```python
from build123d import *

# Parameters (mm, degrees)
F0_R      = 8
F1_DEPTH  = 5
F2_R      = 4
F3_DEPTH  = 6
F4_R      = 1.2
F5_DEPTH  = 9
F6_R      = 5
F7_DEPTH  = 2
F8_R      = 7.5
F8_R_2    = 6.75
F9_DEPTH  = 0.5
F10_SIZE  = 0.2
F11_R     = 0.2
F13_R     = 1.25
F14_DEPTH = 4.5
F15_W     = 2
F15_H     = 12
F16_DEPTH = 1


with BuildPart() as f1:
    # F0 (on Top) → F1 (new body)
    with BuildSketch(Plane.XY):
        Circle(F0_R)
    extrude(amount=F1_DEPTH)

    # F2 (on face) → F3 (join)
    with BuildSketch(Plane(origin=(0, 0, 0), x_dir=(1, 0, 0), z_dir=(0, 0, -1))):
        Circle(F2_R)
    extrude(amount=F3_DEPTH)

    # F4 (on face) → F5 (cut)
    with BuildSketch(Plane(origin=(0, 0, -6), x_dir=(1, 0, 0), z_dir=(0, 0, -1))):
        Circle(F4_R)
    extrude(amount=-F5_DEPTH, mode=Mode.SUBTRACT)

    # F6 (on face) → F7 (cut)
    with BuildSketch(Plane.XY.offset(5)):
        Circle(F6_R)
    extrude(amount=-F7_DEPTH, mode=Mode.SUBTRACT)

    # F8 (on face) → F9 (cut)
    with BuildSketch(Plane.XY.offset(5)):
        Circle(F8_R)
        Circle(F8_R_2, mode=Mode.SUBTRACT)
    extrude(amount=-F9_DEPTH, mode=Mode.SUBTRACT)

    # F10
    f10_edges = [f1.edges().sort_by_distance(p)[0] for p in [
        (-6.75, 0, 5),
    ]]
    chamfer(f10_edges, length=F10_SIZE)

    # F11
    f11_edges = [f1.edges().sort_by_distance(p)[0] for p in [
        (-6.75, 0, 4.8),
        (-1.2, 0, 3),
        (-1.2, 0, -6),
    ]]
    fillet(f11_edges, radius=F11_R)

    # F13 (on Right) → F14 (cut)
    with BuildSketch(Plane.YZ):
        with Locations((0, -3.5)):
            Circle(F13_R)
    extrude(amount=-F14_DEPTH, mode=Mode.SUBTRACT)

    # F15 (on offset) → F16 (cut)
    with BuildSketch(Plane.XY.offset(5)):
        with Locations((7, -0.3699996099)):
            Rectangle(F15_W, F15_H)
    extrude(amount=-F16_DEPTH, mode=Mode.SUBTRACT)


solid = f1.part
```
Can you work these out from the model? Positions are in its coordinate system, mm. A direction names the side the tool comes from. Round coordinates to 2 decimals unless told otherwise and drop trailing zeros. Loops run counter-clockwise (first coordinate to the right, second up) from the corner with the lowest first, then second, coordinate; pieces in that order, holes last.
Item 1: Will these pins go through, and if not, where does the flat tip stop? pin 1 Ø0.6 at (x, y) = (6.5, -1.5) entering from +Z; pin 2 Ø4 at (x, z) = (-2, -1) entering from -Y; pin 3 Ø1 at (x, y) = (0.5, -1.5) entering from +Z.
Item 2: Suppose I cut it at A-A, the plane y = 0. State how many separate pieces and enclosed holes the cut face has, then the cut area to 3 significant figures.
Item 3: Which directions (+Z, -Z, +X, -X, +Y, -Y) give clear straight access to the entire face, cutting with the end or side of a thin tool? Please do faces 1 (the cylindrical face through (-1.08, -4.88, 4.01)), 2 (the flat face through (6, -0.1, 4.5)), 3 (the flat face through (-7.3, -2.3, 5)), 4 (the cylindrical face through (3.695, 1.532, -2.958)), 5 (the cylindrical face through (-2.42, 1.19, -3.12)).
Item 4: Please list where these lines run through material, in increasing order: L1, parallel to X at y = 0, z = -1.5; L2, parallel to Y at x = 0, z = 3.8; L3, parallel to Z at x = -2.7, y = 0.
Item 5: If we mould it in two halves opening along X, with no side actions, what happens to faces 6 (the cylindrical face through (1.145, -0.36, -1.56)), 7 (the flat face through (2, 0, -6)), 8 (the cylindrical face through (-8, 0, 2))? For each: +X half, -X half, draft (parallel to the pull), parting line (faces both ways), or undercut.
Item 6: Suppose I cut it at B-B, the plane z = -3.5. Write out the boundary of the cut face in (x, y).
Reported:
1. pin 1: stops at z = 4
1. pin 2: stops at y = -8
1. pin 3: stops at z = 3
2. separate pieces: 3
2. enclosed holes: 0
2. area: 77.0 mm2
3. face 1: +Z
3. face 2: +Z, +X, +Y, -Y
3. face 3: +Z, +X, -X, +Y, -Y
3. face 4: -Z
3. face 5: -X
4. L1: x = -4 to -1.2, 1.2 to 4
4. L2: y = -8 to -5, 5 to 8
4. L3: z = -6 to -4.75, -2.25 to 3
5. face 6: undercut
5. face 7: draft
5. face 8: parting line
6. outline: (-3.8, -1.25) arc R4 ccw (long way) to (-3.8, 1.25) - (0, 1.25) - (0, 1.2) arc R1.2 cw to (0, -1.2) - (0, -1.25) - close
